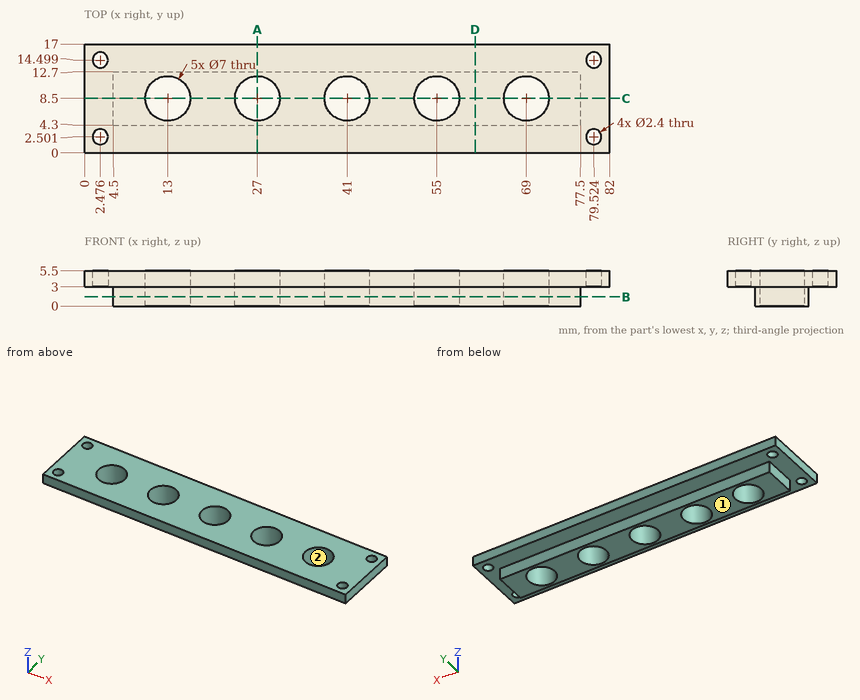
Could you check a few things on this drawing? It's one solid part, dimensions in mm from its lowest x, y, z. Give positions to 0.01 mm unless a question says otherwise; leave off trailing zeros. Loops run counter-clockwise (first coordinate to the right, second up) from the corner with the lowest first, then second, coordinate; pieces in that order, holes last. Notation, with made-up numbers: M 82.25,81 L 119.25,81 A20 ccw 119.25,97 Z; hole C 44,18 d11. An arc over 180 degrees is marked long. One line per question, with ' | ' between items. Start each with the question number.
Q1. If we section it at B-B (z = 1.45): Please give me the cut outline in (x, y).
Q2. If we section it at D-D (x = 61): Please give me the cut outline in (y, z), plus the area to 3 significant figures.
Q3. If we section it at C-C (y = 8.5): Please give me the cut outline in (x, z).
Q4. If we mould it in two halves opening along X, with no side actions, what happens to the marked faces 1 and 2? For each: +X half, -X half, draft (parallel to the pull), parting line (faces both ways), or undercut.
Q5. If I drill on line 1 (X direction, y = 8, z = 2.55); line 2 (X direction, y = 2.25, z = 5.2); line 3 (X direction, y = 7.75, z = 1.6), over which ranges is the centre line in solid material (lowest first)? Write a range as from..to.
Q6. For pin 1 Ø4 at (x, y) = (79.52, 14.5) entering from -Z; pin 2 Ø3 at (y, z) = (6.5, 3.5) entering from -X; pin 3 Ø1.5 at (y, z) = (8, 1) entering from +X; pin 4 Ø1.5 at (y, z) = (9.5, 1.5) entering from -X, each with a flat end and sliding along its axis, tell me the tip position at first contact or that it passes through.
Q7. If we section it at A-A (x = 27): Please give me the cut outline in (y, z).
Computed:
1) outline: M 4.5,4.3 L 77.5,4.3 L 77.5,12.7 L 4.5,12.7 Z; hole C 13,8.5 d7; hole C 27,8.5 d7; hole C 41,8.5 d7; hole C 55,8.5 d7; hole C 69,8.5 d7
2) outline: M 0,3 L 4.3,3 L 4.3,0 L 12.7,0 L 12.7,3 L 17,3 L 17,5.5 L 0,5.5 Z | area: 67.7 mm²
3) outline: M 0,3 L 4.5,3 L 4.5,0 L 9.5,0 L 9.5,5.5 L 0,5.5 Z; M 16.5,0 L 23.5,0 L 23.5,5.5 L 16.5,5.5 Z; M 30.5,0 L 37.5,0 L 37.5,5.5 L 30.5,5.5 Z; M 44.5,0 L 51.5,0 L 51.5,5.5 L 44.5,5.5 Z; M 58.5,0 L 65.5,0 L 65.5,5.5 L 58.5,5.5 Z; M 72.5,0 L 77.5,0 L 77.5,3 L 82,3 L 82,5.5 L 72.5,5.5 Z
4) face 1: draft | face 2: undercut
5) line 1: x = 4.5..9.54, 16.46..23.54, 30.46..37.54, 44.46..51.54, 58.46..65.54, 72.46..77.5 | line 2: x = 0..1.3, 3.65..78.35, 80.7..82 | line 3: x = 4.5..9.58, 16.42..23.58, 30.42..37.58, 44.42..51.58, 58.42..65.58, 72.42..77.5
6) pin 1: stops at z = 3 | pin 2: stops at x = 0 | pin 3: stops at x = 77.5 | pin 4: stops at x = 4.5
7) outline: M 0,3 L 4.3,3 L 4.3,0 L 5,0 L 5,5.5 L 0,5.5 Z; M 12,0 L 12.7,0 L 12.7,3 L 17,3 L 17,5.5 L 12,5.5 Z
